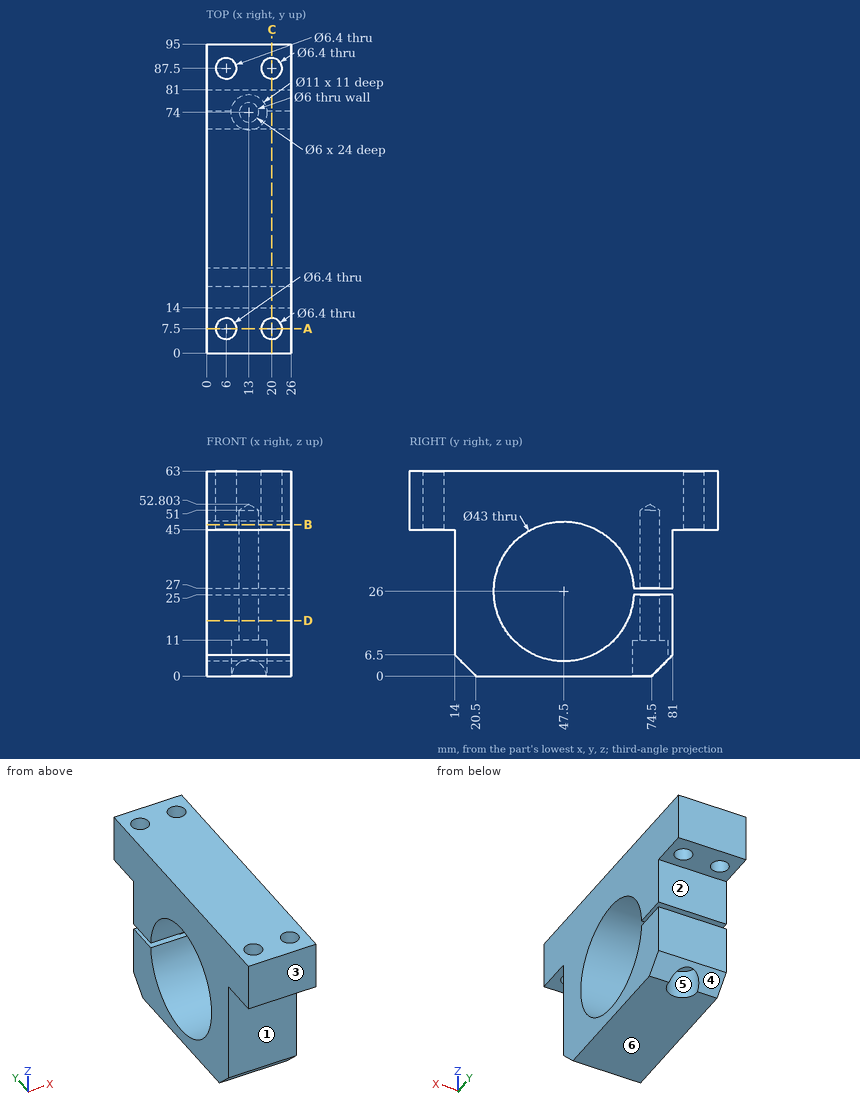
Could you check a few things on this drawing? It's one solid part, dimensions in mm from its lowest x, y, z. A direction names the side the tool comes from. Coordinates: 2 decimals unless noted, no trailing zeros. Order: outer loops, then holes, each group sorted by start corner. A loop starts at its lowest first (then second) coordinate and runs counter-clockwise, first axis right, second up.
1. For the marked faces 1, 2 and 3, which set-ups out of +Z, -Z, +X, -X, +Y, -Y let a thin tool reach every point of the face, with its end or its side?
2. If we section it at C-C (x = 20): Please give me the cut outline in (y, z).
3. I'm going to push flat-ended pins straight in: pin 1 (10 mm diameter, centred on x = 6, y = 87.5, fed in from -Z); pin 2 (8 mm diameter, centred on y = 36.5, z = 13.5, fed in from -X); pin 3 (1.5 mm diameter, centred on x = 19, z = 23, fed in from +Y); pin 4 (5 mm diameter, centred on x = 12.5, z = 32.5, fed in from -Y). Where does each tip first touch, or does it pass through?
4. If we section it at A-A (y = 7.5): Please give me the cut outline in (x, z).
5. I need wall thicknesses on line 1 (Y direction, x = 20, z = 59); line 2 (Z direction, x = 9, y = 76); line 3 (Z direction, x = 5.5, y = 70.5). Which ranges of each line are inside material? Lowest first, please.
6. If we section it at B-B (z = 46.5): Please give me the cut outline in (x, y).
7. Thinking about a two-plate mould opening in Y: for the marked faces 4, 5 and 6, which applies, +Y half, -Y half, draft (parallel to the pull), parting line (faces both ways), or undercut?
8. If we section it at D-D (z = 17): Please give me the cut outline in (x, y) (1 decimal).
Entries:
1. face 1: -Z, +X, -X, -Y
1. face 2: -Z, +X, -X, +Y
1. face 3: +Z, -Z, +X, -X, -Y
2. outline: (0, 45) - (4.3, 45) - (4.3, 63) - (0, 63) - close; (10.7, 45) - (14, 45) - (14, 6.5) - (20.5, 0) - (74.5, 0) - (81, 6.5) - (81, 25) - (68.98, 25) arc R21.5 cw (long way) to (68.98, 27) - (81, 27) - (81, 45) - (84.3, 45) - (84.3, 63) - (10.7, 63) - close; (90.7, 45) - (95, 45) - (95, 63) - (90.7, 63) - close
3. pin 1: stops at z = 45
3. pin 2: passes through
3. pin 3: stops at y = 81
3. pin 4: stops at y = 14
4. outline: (0, 45) - (2.8, 45) - (2.8, 63) - (0, 63) - close; (9.2, 45) - (16.8, 45) - (16.8, 63) - (9.2, 63) - close; (23.2, 45) - (26, 45) - (26, 63) - (23.2, 63) - close
5. line 1: y = 0 to 4.3, 10.7 to 84.3, 90.7 to 95
5. line 2: z = 11 to 25, 27 to 63
5. line 3: z = 0 to 25, 27 to 63
6. outline: (0, 0) - (26, 0) - (26, 41.02) - (0, 41.02) - close; (0, 53.98) - (26, 53.98) - (26, 95) - (0, 95) - close; hole circle Ø6.4 at (6, 7.5); hole circle Ø6.4 at (6, 87.5); hole circle Ø6 at (13, 74); hole circle Ø6.4 at (20, 7.5); hole circle Ø6.4 at (20, 87.5)
7. face 4: +Y half
7. face 5: undercut
7. face 6: draft
8. outline: (0, 14) - (26, 14) - (26, 28) - (0, 28) - close; (0, 67) - (26, 67) - (26, 81) - (0, 81) - close; hole circle Ø6 at (13, 74)
